Part model, mm, in its own coordinate system. Face numbers are marked on the shaded views. A direction names the side the tool comes from. Round coordinates to 2 decimals unless told otherwise and drop trailing zeros. Loops run counter-clockwise (first coordinate to the right, second up) from the corner with the lowest first, then second, coordinate; pieces in that order, holes last. Notation, with made-up numbers: M 19.25,-12 L 46.25,-12 A23 cw 46.25,2 Z; hole C 27,69.25 d1. An arc over 180 degrees is marked long. Answer as CSV lines item,"result". Start each with the question number.
Item 1: Drop flat-ended pins along their axis: pin 1 Ø2 at (x, z) = (0, 29.5) entering from +Y; pin 2 Ø1.5 at (y, z) = (0.5, 29) entering from +X; pin 3 Ø4.5 at (x, z) = (-1, -3) entering from +Y. Give the stop position or say it passes through.
Item 2: Band-saw the part on B-B (y = -3.75). Give the cut face in (x, z).
Item 3: Band-saw the part on D-D (x = -4.5). Give the cut face in (y, z).
Item 4: Wall check: line 1 (Z direction, x = -6.25, y = -0.5); line 2 (Z direction, x = -3.5, y = -5.75); line 3 (Y direction, x = -3, z = -4). Give the ranges that are in metal, low to high.
Item 5: Which spindle directions (+Z, -Z, +X, -X, +Y, -Y) get a long thin tool onto all of the face, cutting with end or side? Do the marked faces 1, 2, 3 and 4. Say none if no direction does.
Item 6: Band-saw the part on C-C (z = 27.5). Give the cut face in (x, y), and give its area (3 significant figures).
Item 7: Band-saw the part on A-A (x = -1.5). Give the cut face in (y, z), and give its area (3 significant figures).
```python
from build123d import *

# Parameters (mm, degrees)
F0_W     = 17.526
F0_H     = 23.114
F1_DEPTH = 26.416
F2_W     = 9.906
F2_H     = 5.056186
F3_DEPTH = 6.858
F4_W     = 7.9375
F4_H     = 11.1125
F5_DEPTH = 5.334


with BuildPart() as f1:
    # F0 (on Top) → F1 (new body)
    with BuildSketch(Plane.XY):
        Rectangle(F0_W, F0_H)
    extrude(amount=F1_DEPTH)

    # F2 (on face) → F3 (join)
    with BuildSketch(Plane.XY.offset(26.416)):
        Rectangle(F2_W, F2_H)
    extrude(amount=F3_DEPTH)

    # F4 (on face) → F5 (join)
    with BuildSketch(Plane(origin=(0, 0, 0), x_dir=(1, 0, 0), z_dir=(0, 0, -1))):
        with Locations((0, 6.00075)):
            Rectangle(F4_W, F4_H)
    extrude(amount=F5_DEPTH)


solid = f1.part
```
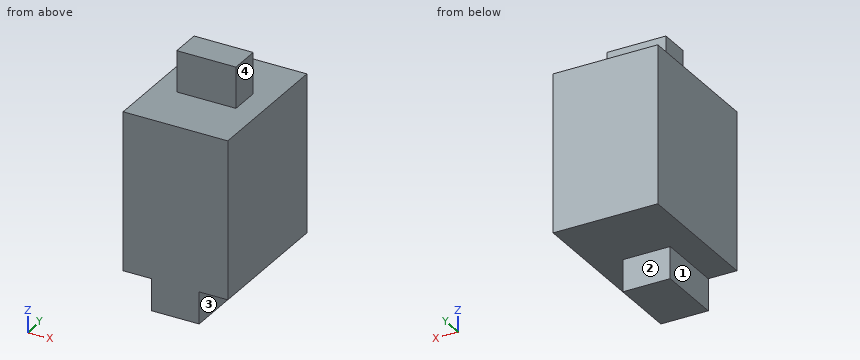
Answer block:
1,pin 1,"stops at y = 2.53"
1,pin 2,"stops at x = 4.95"
1,pin 3,"stops at y = -0.44"
2,outline,"M -8.76,0 L -3.97,0 L -3.97,-5.33 L 3.97,-5.33 L 3.97,0 L 8.76,0 L 8.76,26.42 L -8.76,26.42 Z"
3,outline,"M -11.56,0 L 11.56,0 L 11.56,26.42 L 2.53,26.42 L 2.53,33.27 L -2.53,33.27 L -2.53,26.42 L -11.56,26.42 Z"
4,line 1,"z = 0 to 26.42"
4,line 2,"z = -5.33 to 26.42"
4,line 3,"y = -11.56 to -0.44"
5,face 1,"-Z, -X, +Y, -Y"
5,face 2,"-Z, +X, -X, +Y"
5,face 3,"-Z, +X, +Y, -Y"
5,face 4,"+Z, +X, +Y, -Y"
6,outline,"M -4.95,-2.53 L 4.95,-2.53 L 4.95,2.53 L -4.95,2.53 Z"
6,area,"50.1 mm^2"
7,outline,"M -11.56,-5.33 L -0.44,-5.33 L -0.44,0 L 11.56,0 L 11.56,26.42 L 2.53,26.42 L 2.53,33.27 L -2.53,33.27 L -2.53,26.42 L -11.56,26.42 Z"
7,area,"705 mm^2"
